Check sheet for the drawn part. Datum: minimum x, y, z corner. Units: mm. A direction names the side the tool comes from. Round coordinates to 2 decimals unless told otherwise and drop trailing zeros. Write each loop counter-clockwise with the first axis right and the second up, starting at its lowest first coordinate (ties: lowest second). Pieces come first, ordered by that corner, then holes. Notation, with made-up numbers: (77, 23.25) - (99, 23.25) arc R11 cw to (99, 43.25) - close; hole circle Ø2 at (68, 10.5). An arc over 180 degrees is marked (long way). Answer as a JSON object with one key per item and string values. Group by question number.
Item 1: Release check for a two-part mould opening along X. For the marked faces 1, 2 and 3 record: pulls with the +X half, pulls with the -X half, needs draft (parallel to the pull), parting line crosses it, or undercut.
Item 2: Sectioned sample at B-B on z = 60. Record the boundary of the cut face in (x, y), plus the area to 3 significant figures.
Item 3: Thickness scan on line 1 (Z direction, x = 15, y = 5.5); line 2 (Z direction, x = 19.5, y = 4.25) (1 decimal); line 3 (Z direction, x = 28.5, y = 4.25) (1 decimal). Record the ranges inside material, lowest first.
Item 4: Gauge pin test, flat ends, axial feed: P1, Ø13.5, axis at x = 15, z = 60, coming from the -Y side; P2, Ø5, axis at y = 7, z = 59.5, coming from the -X side; P3, Ø2.5, axis at x = 28.5, y = 5, coming from the -Z side (3 decimals); P4, Ø5, axis at x = 15, z = 10, coming from the +Y side. Record the tip position at first contact, or that the pin passes through.
Item 5: Set-up check for the marked faces 4, 5, 6, 7 and 8: record each of +Z, -Z, +X, -X, +Y, -Y from which the full face is reachable in a straight line by a thin tool's end or side.
Item 6: Sectioned sample at A-A on y = 2.25. Count the separate pieces of the cut face and the enclosed holes in it, plus the area to 3 significant figures.
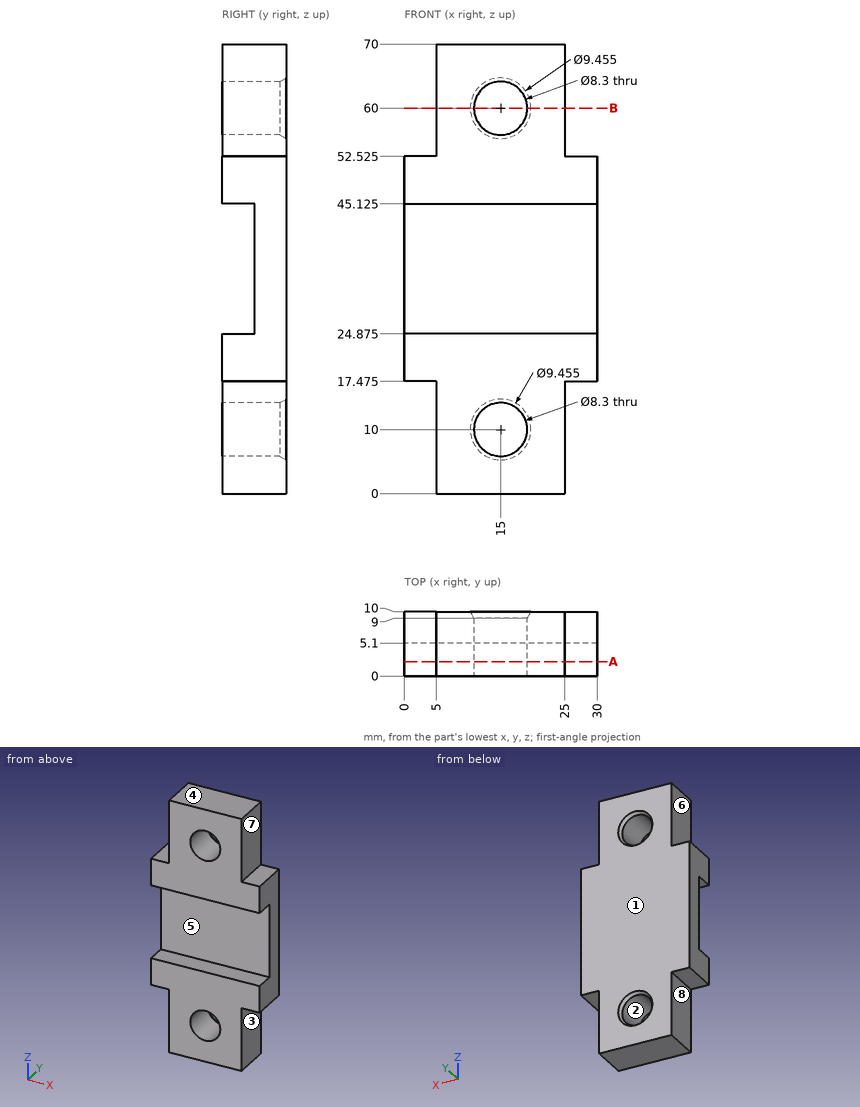
Completed:
{
 "1": {"face 1": "needs draft", "face 2": "undercut", "face 3": "pulls with the +X half"},
 "2": {"outline": "(5, 0) - (10.85, 0) - (10.85, 9) - (10.27, 10) - (5, 10) - close; (19.15, 0) - (25, 0) - (25, 10) - (19.73, 10) - (19.15, 9) - close", "area": "116 mm²"},
 "3": {"line 1": "0 to 5.85, 14.15 to 55.85, 64.15 to 70", "line 2": "0 to 24.9, 45.1 to 70", "line 3": "17.5 to 24.9, 45.1 to 52.5"},
 "4": {"P1": "y = 0", "P2": "x = 5", "P3": "z = 17.475", "P4": "through"},
 "5": {"face 4": "+Z, +X, -X, +Y, -Y", "face 5": "+X, -X, -Y", "face 6": "+Z, -X, +Y, -Y", "face 7": "+Z, +X, +Y, -Y", "face 8": "-Z, -X, +Y, -Y"},
 "6": {"separate pieces": "2", "enclosed holes": "2", "area": "1,030 mm²"}
}
